For this review, take the finished solid that the model builds, in its own axes (mm). Face numbers are marked on the shaded views. Round coordinates to 2 decimals unless told otherwise and drop trailing zeros. Write each loop counter-clockwise with the first axis right and the second up, starting at its lowest first coordinate (ties: lowest second). Pieces come first, ordered by that corner, then holes. Notation, with made-up numbers: M -40,0.25 L -17,0.25 A15 ccw -17,12.25 Z; hole C 8,-34.75 d7. An arc over 180 degrees is marked long. Use one line per item in the form item = value. Start each with the question number.
Item 1: Draft analysis for pull direction Z (two halves, no side actions). For the marked faces 1, 2 and 3, state which applies: released by +Z, released by -Z, zero draft, split by the parting line, or undercut.
Item 2: For line 1 (Z direction, x = 0, y = 17.8); line 2 (X direction, y = 13.5, z = 16.75), list the stretches that pass through material, from the lowest coordinate up. Write a range as [from, to].
Item 3: Add section B-B (z = 17.5). State the section outline as (x, y) points, and give its area (3 significant figures).
Item 4: Add section A-A (x = 0). State the section outline as (y, z) points.
Item 5: For P1, Ø3, axis at y = 16.5, z = 15.5, coming from the -X side; P2, Ø1.7, axis at x = 0, z = 13.41, coming from the -Y side, all flat-tipped, find the tip position at first contact; note any pin that passes through.
from build123d import *

# Parameters (mm, degrees)
SKETCH2_R    = 16.7005
SKETCH2_R_2  = 15.0495
SCALE1_SCALE = 0.095238095


with BuildPart() as part:
    # Sweep1: sweep along a path in Sketch1
    with BuildLine(Plane(origin=(0, 0, 0), x_dir=(0, 0, -1), z_dir=(1, 0, 0))) as sweep1_path:
        Line((-50.8, 0), (-38.1, 0))
        ThreePointArc((-38.1, 0), (-11.159231637, 11.159231637), (0, 38.1))
        Line((0, 38.1), (0, 50.8))
    # Sketch2 → Sweep1 (sweep)
    with BuildSketch(Plane.XY.offset(50.8)):
        Circle(SKETCH2_R)
        Circle(SKETCH2_R_2, mode=Mode.SUBTRACT)
    sweep(path=sweep1_path.line)

    # Sketch3 → Cut-Revolve1 (revolve, cut)
    with BuildSketch(Plane(origin=(0, 0, 0), x_dir=(0, 1, 0), z_dir=(-1, 0, 0))):
        Polygon((-16.7005, -50.8), (-16.7005, -50.14220894), (-15.84325, -50.8), align=None)
    revolve(axis=Axis((0, 0, 50.8), (0, 0, -1)), mode=Mode.SUBTRACT)

    # Sketch3<4> → Cut-Revolve2 (revolve, cut)
    with BuildSketch(Plane(origin=(0, 0, 0), x_dir=(0, 1, 0), z_dir=(-1, 0, 0))):
        Polygon((50.8, 15.84325), (50.8, 16.7005), (50.14220894, 16.7005), align=None)
    revolve(axis=Axis((0, 50.8, 0), (0, -1, 0)), mode=Mode.SUBTRACT)


with BuildPart() as part_1:
    # Scale1: scaled about (0, 14.816195429, 14.816195429)
    add(part.part.scale(SCALE1_SCALE).moved(Location((0, 13.405129198, 13.405129198))))


solid = part_1.part
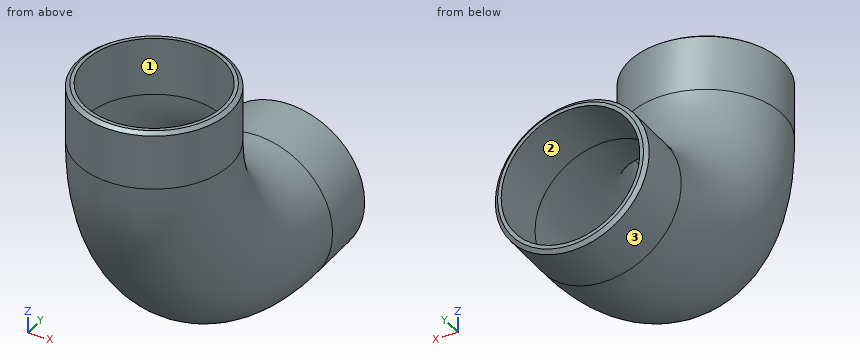
Calculated:
q1.face_1 = zero draft
q1.face_2 = undercut
q1.face_3 = split by the parting line
q2.line_1 = [11.81, 11.97], [14.84, 15]
q2.line_2 = [-1.59, -1.43], [1.43, 1.59]
q3.outline = C 0,13.41 d3.18; hole C 0,13.41 d2.87
q3.area = 1.49 mm^2
q4.outline = M 11.81,17.03 A5.22 ccw 17.03,11.81 L 18.18,11.81 L 18.24,11.9 L 18.24,11.97 L 17.03,11.97 A5.06 cw 11.97,17.03 L 11.97,18.24 L 11.9,18.24 L 11.81,18.18 Z; M 14.84,17.03 A2.2 ccw 17.03,14.84 L 18.24,14.84 L 18.24,14.91 L 18.18,15 L 17.03,15 A2.04 cw 15,17.03 L 15,18.18 L 14.91,18.24 L 14.84,18.24 Z
q5.P1 = -1.51
q5.P2 = 12.61
